from build123d import *


with BuildPart() as part:
    # Sketch1 → Revolve2 (revolve)
    with BuildSketch(Plane.XY, mode=Mode.PRIVATE) as revolve2_sk:
        with BuildLine():
            Line((11, 4.25), (11, 1.5))
            ThreePointArc((11, 1.5), (10.5, 0), (11, -1.5))
            Line((11, -1.5), (11, -4.25))
            Line((11, -4.25), (10.5, -4.25))
            Line((10.5, -4.25), (10.5, -5))
            Line((10.5, -5), (8.5, -5))
            Line((8.5, -5), (8.5, 5))
            Line((8.5, 5), (10.5, 5))
            Line((10.5, 5), (10.5, 4.25))
            Line((10.5, 4.25), (11, 4.25))
        make_face()
    revolve(revolve2_sk.sketch.rotate(Axis((0, 0, 0), (0, 1, 0)), 90), axis=Axis((0, 0, 0), (0, 1, 0)))


solid = part.part
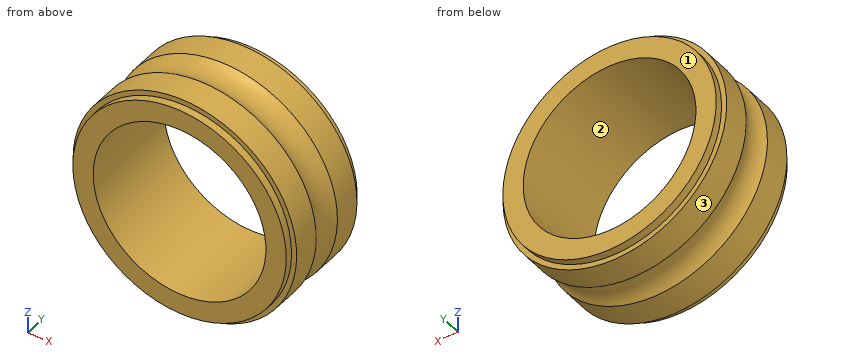
Here's how the part is built. I have some questions about the finished solid (model axes, mm). Face numbers are marked on the shaded views. Coordinates: 2 decimals unless noted, no trailing zeros. Write each loop counter-clockwise with the first axis right and the second up, starting at its lowest first coordinate (ties: lowest second). Pieces come first, ordered by that corner, then holes. Notation, with made-up numbers: (-36, 33) - (8, 33) arc R26 cw to (8, 67) - close; hole circle Ø10 at (9, 17.25). An arc over 180 degrees is marked (long way). Use one line per item in the form item = value.
1) Suppose I cut it at D-D, the plane y = -0.5. Write out the boundary of the cut face in (x, z).
Solved:
outline = circle Ø21.1 at (0, 0); hole circle Ø17 at (0, 0)
2) Thinking about a two-plate mould opening in X: for the marked faces 1, 2 and 3, which applies, released by +X, released by -X, zero draft, split by the parting line, or undercut?
Solved:
face_1 = zero draft
face_2 = undercut
face_3 = split by the parting line
3) I need wall thicknesses on line 1 (X direction, y = -3, z = 0); line 2 (Y direction, x = 9.25, z = 5.75); line 3 (X direction, y = 0.5, z = -0.75). Which ranges of each line are inside material? Lowest first, please.
Solved:
line_1 = -11 to -8.5, 8.5 to 11
line_2 = -4.25 to -1.34, 1.34 to 4.25
line_3 = -10.52 to -8.47, 8.47 to 10.52
4) Suppose I cut it at A-A, the plane x = 0. Write out the boundary of the cut face in (y, z).
Solved:
outline = (-5, -10.5) - (-4.25, -10.5) - (-4.25, -11) - (-1.5, -11) arc R2.5 cw to (1.5, -11) - (4.25, -11) - (4.25, -10.5) - (5, -10.5) - (5, -8.5) - (-5, -8.5) - close; (-5, 8.5) - (5, 8.5) - (5, 10.5) - (4.25, 10.5) - (4.25, 11) - (1.5, 11) arc R2.5 cw to (-1.5, 11) - (-4.25, 11) - (-4.25, 10.5) - (-5, 10.5) - close
5) I'm going to push flat-ended pins straight in: P1, Ø5, axis at y = -4, z = -4, coming from the +X side; P2, Ø5, axis at x = -6, y = 2, coming from the -Z side; P3, Ø2, axis at x = 5, y = -0.5, coming from the -Z side. Where does each tip first touch, or does it pass through?
Solved:
P1 = 10.9
P2 = -10.43
P3 = -9.94
6) Suppose I cut it at B-B, the plane z = 0. Write out the boundary of the cut face in (x, y).
Solved:
outline = (-11, -4.25) - (-10.5, -4.25) - (-10.5, -5) - (-8.5, -5) - (-8.5, 5) - (-10.5, 5) - (-10.5, 4.25) - (-11, 4.25) - (-11, 1.5) arc R2.5 cw to (-11, -1.5) - close; (8.5, -5) - (10.5, -5) - (10.5, -4.25) - (11, -4.25) - (11, -1.5) arc R2.5 cw to (11, 1.5) - (11, 4.25) - (10.5, 4.25) - (10.5, 5) - (8.5, 5) - close
7) Suppose I cut it at C-C, the plane y = -3.5. Write out the boundary of the cut face in (x, z), plus the area to 3 significant figures.
Solved:
outline = circle Ø22 at (0, 0); hole circle Ø17 at (0, 0)
area = 153 mm2
